Can you work these out from the model? Positions are in its coordinate system, mm. Give positions to 0.01 mm unless a question says otherwise; leave off trailing zeros. Order: outer loops, then holes, each group sorted by start corner. A loop starts at its lowest first (then second) coordinate and runs counter-clockwise, first axis right, second up.
Item 1: If we mould it in two halves opening along X, with no side actions, what happens to faces 1 (the flat face through (-9, 1, 5)), 2 (the flat face through (13.84, 1, 0)), 3 (the cylindrical face through (10.082, 1.014, -0.273))? For each: +X half, -X half, draft (parallel to the pull), parting line (faces both ways), or undercut.
Item 2: I want a section at A-A, the plane x = 8. Write out the boundary of the cut face in (y, z).
Item 3: I'm going to push a flat-ended pin straight in: pin 1 Ø2.5 at (x, z) = (8, 0) entering from +Y. Where does the tip first touch, or does it pass through?
Item 4: I want a section at C-C, the plane z = 0. Write out the boundary of the cut face in (x, y).
Item 5: I want a section at B-B, the plane y = 1.55. Write out the boundary of the cut face in (x, z), then the cut area to 3 significant figures.
Item 6: If I drill on line 1 along X through (y, z) = (0.85, 0); line 2 along X through (y, z) = (0.5, -0.5); line 3 along X through (y, z) = (1.5, 3), over which ranges is the centre line in solid material (lowest first)?
Item 7: I want a section at D-D, the plane z = 3. Write out the boundary of the cut face in (x, y).
```python
from build123d import *

# Parameters (mm, degrees)
SKETCH1_W           = 27.68
SKETCH1_H           = 10
BOSS_EXTRUDE1_DEPTH = 2
CUT_EXTRUDE1_REACH  = 16.851
SKETCH2_R           = 2.1
CUT_EXTRUDE2_REACH  = 16.851
SKETCH3_R           = 4.5


with BuildPart() as part:
    # Sketch1 → Boss-Extrude1 (new body)
    with BuildSketch(Plane(origin=(0, 0, 0), x_dir=(1, 0, 0), z_dir=(0, 1, 0))):
        Rectangle(SKETCH1_W, SKETCH1_H)
    extrude(amount=BOSS_EXTRUDE1_DEPTH)

    # Sketch2 → Cut-Extrude1 (cut, up to next)
    with BuildSketch(Plane(origin=(0, 2, 0), x_dir=(1, 0, 0), z_dir=(0, 1, 0)), mode=Mode.PRIVATE) as cut_extrude1_sk1:
        with Locations(Location((8, 0, 0), (0, 0, 270))):
            Circle(SKETCH2_R)
    cut_extrude1_tool1 = extrude(cut_extrude1_sk1.sketch, amount=-CUT_EXTRUDE1_REACH, mode=Mode.PRIVATE) & part.part
    # Sketch2 → Cut-Extrude1 (cut, up to next)
    with BuildSketch(Plane(origin=(0, 2, 0), x_dir=(1, 0, 0), z_dir=(0, 1, 0)), mode=Mode.PRIVATE) as cut_extrude1_sk2:
        with Locations(Location((-8, 0, 0), (0, 0, 270))):
            Circle(SKETCH2_R)
    cut_extrude1_tool2 = extrude(cut_extrude1_sk2.sketch, amount=-CUT_EXTRUDE1_REACH, mode=Mode.PRIVATE) & part.part
    add(cut_extrude1_tool1.solids().sort_by_distance((8, 2, 0))[0], mode=Mode.SUBTRACT)
    add(cut_extrude1_tool2.solids().sort_by_distance((-8, 2, 0))[0], mode=Mode.SUBTRACT)

    # Sketch3 → Cut-Extrude2 (cut, up to next)
    with BuildSketch(Plane.XZ, mode=Mode.PRIVATE) as cut_extrude2_sk1:
        with Locations((0, 7)):
            Circle(SKETCH3_R)
    cut_extrude2_tool1 = extrude(cut_extrude2_sk1.sketch, amount=-CUT_EXTRUDE2_REACH, mode=Mode.PRIVATE) & part.part
    add(cut_extrude2_tool1.solids().sort_by_distance((0, 0, 7))[0], mode=Mode.SUBTRACT)


solid = part.part
```
Results list:
1. face 1: draft
1. face 2: +X half
1. face 3: undercut
2. outline: (0, -5) - (2, -5) - (2, -2.1) - (0, -2.1) - close; (0, 2.1) - (2, 2.1) - (2, 5) - (0, 5) - close
3. pin 1: passes through
4. outline: (-13.84, 0) - (-10.1, 0) - (-10.1, 2) - (-13.84, 2) - close; (-5.9, 0) - (5.9, 0) - (5.9, 2) - (-5.9, 2) - close; (10.1, 0) - (13.84, 0) - (13.84, 2) - (10.1, 2) - close
5. outline: (-13.84, -5) - (13.84, -5) - (13.84, 5) - (4.03, 5) arc R4.5 cw to (-4.03, 5) - (-13.84, 5) - close; hole circle Ø4.2 at (-8, 0); hole circle Ø4.2 at (8, 0)
5. area: 235 mm2
6. line 1: x = -13.84 to -10.1, -5.9 to 5.9, 10.1 to 13.84
6. line 2: x = -13.84 to -10.04, -5.96 to 5.96, 10.04 to 13.84
6. line 3: x = -13.84 to -2.06, 2.06 to 13.84
7. outline: (-13.84, 0) - (-2.06, 0) - (-2.06, 2) - (-13.84, 2) - close; (2.06, 0) - (13.84, 0) - (13.84, 2) - (2.06, 2) - close
